Model file for the job. Use its own axes, mm. Face numbers are marked on the shaded views. A direction names the side the tool comes from. Round coordinates to 2 decimals unless told otherwise and drop trailing zeros. Loops run counter-clockwise (first coordinate to the right, second up) from the corner with the lowest first, then second, coordinate; pieces in that order, holes last. Notation, with made-up numbers: M 43,78.25 L 60,78.25 A36 ccw 60,112.25 Z; hole C -18,48.25 d11. An arc over 180 degrees is marked long. Answer in a Markdown table with one row per item.
Autodesk Inventor part; units mm, degrees
ref_plane "YZ Plane" through (0, 0, 0) normal (1, 0, 0) x (0, 1, 0)
ref_plane "XZ Plane" through (0, 0, 0) normal (0, 1, 0) x (-1, 0, 0)
ref_plane "XY Plane" through (0, 0, 0) normal (0, 0, 1) x (1, 0, 0)
sketch "Sketch1" plane through (0, 0, 0) normal (0, 1, 0) x (-1, 0, 0)
  circle A0 centre (0, 0) radius 1.25
  circle A1 centre (0, 0) radius 1.75
  dimension "d0" = 2.5
  dimension "d1" = 3.5
extrude "Extrusion1" add sketch "Sketch1" along normal blind 2
sketch "Sketch2" plane through (0, 0, 0) normal (0, -1, 0) x (1, 0, 0)
  circle A0 centre (0, 0) radius 1.75
extrude "Extrusion2" add sketch "Sketch2" along normal blind 0.5
sketch "Sketch3" plane through (0, 0, 0) normal (0, 1, 0) x (1, 0, 0)
  circle A0 centre (0, 0) radius 0.75
  dimension "d6" = 1.5
extrude "Extrusion3" add sketch "Sketch3" along normal blind 3.7
sketch "Sketch4" plane through (0, -0.5, 0) normal (0, -1, 0) x (1, 0, 0)
  circle A0 centre (0, 0) radius 0.75
  circle A1 centre (0, 0) radius 0.75
extrude "Extrusion4" add sketch "Sketch4" along normal blind 11.75
properties part number "plunger extension" material "ABS Plastic"
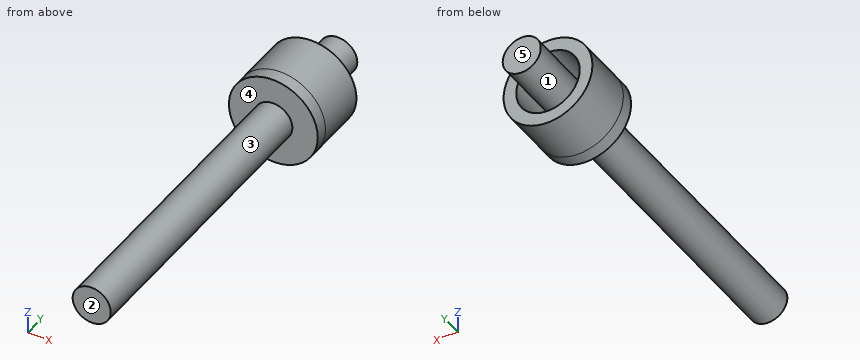
1. Wall check: probe 1 along Z at (x, y) = (0, 0.85); probe 2 along Y at (x, z) = (-0.8, -1.1); probe 3 along Y at (x, z) = (-0.75, 0.4). Give the ranges that are in metal, low to high.
Verdict:
| item | result |
|---|---|
| probe 1 | z = -1.75 to -1.25, -0.75 to 0.75, 1.25 to 1.75 |
| probe 2 | y = -0.5 to 2 |
| probe 3 | y = -0.5 to 0 |
2. Mould opens along X. For the marked faces 1, 2 and 3 say: +X half, -X half, draft (parallel to the pull), parting line (faces both ways), or undercut.
Verdict:
| item | result |
|---|---|
| face 1 | undercut |
| face 2 | draft |
| face 3 | parting line |
3. Tool access for the marked faces 4 and 5: list every direction of +Z, -Z, +X, -X, +Y, -Y with a clear straight run to the whole face (end or side of a thin tool).
Verdict:
| item | result |
|---|---|
| face 4 | -Y |
| face 5 | +Z, -Z, +X, -X, +Y |
4. Saw through at A-A (y = 1). Write the cut outline in (x, z).
Verdict:
| item | result |
|---|---|
| outline | C 0,0 d3.5; C 0,0 d1.5; hole C 0,0 d2.5 |
5. Saw through at C-C (z = 0). Write the cut outline in (x, y), and give its area (3 significant figures).
Verdict:
| item | result |
|---|---|
| outline | M -1.75,-0.5 L -0.75,-0.5 L -0.75,-12.25 L 0.75,-12.25 L 0.75,-0.5 L 1.75,-0.5 L 1.75,2 L 1.25,2 L 1.25,0 L 0.75,0 L 0.75,3.7 L -0.75,3.7 L -0.75,0 L -1.25,0 L -1.25,2 L -1.75,2 Z |
| area | 26.9 mm² |
6. Saw through at B-B (x = 0). Write the cut outline in (y, z), and give its area (3 significant figures).
Verdict:
| item | result |
|---|---|
| outline | M -12.25,-0.75 L -0.5,-0.75 L -0.5,-1.75 L 2,-1.75 L 2,-1.25 L 0,-1.25 L 0,-0.75 L 3.7,-0.75 L 3.7,0.75 L 0,0.75 L 0,1.25 L 2,1.25 L 2,1.75 L -0.5,1.75 L -0.5,0.75 L -12.25,0.75 Z |
| area | 26.9 mm² |
7. Saw through at D-D (y = -3.5). Write the cut outline in (x, z), and give its area (3 significant figures).
Verdict:
| item | result |
|---|---|
| outline | C 0,0 d1.5 |
| area | 1.77 mm² |
